Verification items for the finished model (mm, model axes). A direction names the side the tool comes from. Round coordinates to 2 decimals unless told otherwise and drop trailing zeros. Write each loop counter-clockwise with the first axis right and the second up, starting at its lowest first coordinate (ties: lowest second). Pieces come first, ordered by that corner, then holes. Notation, with made-up numbers: (51, 6.25) - (95, 6.25) arc R28 ccw to (95, 31.25) - close; hole circle Ø2 at (60, -6). An arc over 180 degrees is marked (long way). Answer as a JSON object with one key per item and string values.
```python
from build123d import *

# Parameters (mm, degrees)
BOSS_EXTRUDE1_DEPTH = 2.54
SKETCH6_W           = 5
SKETCH6_H           = 2.5
CUT_EXTRUDE2_DEPTH  = 0.2


with BuildPart() as part:
    # Sketch3 → Boss-Extrude1 (new body)
    with BuildSketch(Plane(origin=(0, 0, 0), x_dir=(1, 0, 0), z_dir=(0, 1, 0))):
        with BuildLine():
            ThreePointArc((-91.6492325, -96.833825344), (-94.514268143, 0.78027625), (-91.6492325, 98.394377843))
            ThreePointArc((-91.6492325, 98.394377843), (-77.728790436, 116.300836492), (-57.46959223, 126.498133029))
            ThreePointArc((-57.46959223, 126.498133029), (0, 128.705492461), (57.46959223, 126.498133029))
            ThreePointArc((57.46959223, 126.498133029), (77.728790436, 116.300836492), (91.6492325, 98.394377843))
            ThreePointArc((91.6492325, 98.394377843), (94.514268143, 0.78027625), (91.6492325, -96.833825344))
            ThreePointArc((91.6492325, -96.833825344), (77.728790436, -114.740283992), (57.46959223, -124.937580529))
            ThreePointArc((57.46959223, -124.937580529), (0, -127.144939961), (-57.46959223, -124.937580529))
            ThreePointArc((-57.46959223, -124.937580529), (-77.728790436, -114.740283992), (-91.6492325, -96.833825344))
        make_face()
    extrude(amount=BOSS_EXTRUDE1_DEPTH)

    # Sketch6 → Cut-Extrude2 (cut)
    with BuildSketch(Plane.XZ):
        Polygon((-80.884003768, 97.161784557), (-83.675257034, 101.310146306), (-81.601076159, 102.705772939), (-78.809822893, 98.55741119), align=None)
        Polygon((-60.2566864, 111.041014588), (-63.047939666, 115.189376338), (-65.122120541, 113.793749705), (-62.330867275, 109.645387955), align=None)
        Polygon((-67.644809829, 81.963964192), (-69.718990703, 80.568337559), (-72.510243969, 84.716699309), (-70.436063095, 86.112325942), align=None)
        Polygon((-51.16585421, 93.051940957), (-49.091673336, 94.44756759), (-51.882926602, 98.59592934), (-53.957107476, 97.200302707), align=None)
        Polygon((51.882926602, 98.59592934), (53.957107476, 97.200302707), (51.16585421, 93.051940957), (49.091673336, 94.44756759), align=None)
        Polygon((65.122120541, 113.793749705), (62.330867275, 109.645387955), (60.2566864, 111.041014588), (63.047939666, 115.189376338), align=None)
        Polygon((67.644809829, 81.963964192), (69.718990703, 80.568337559), (72.510243969, 84.716699309), (70.436063095, 86.112325942), align=None)
        Polygon((80.884003768, 97.161784557), (83.675257034, 101.310146306), (81.601076159, 102.705772939), (78.809822893, 98.55741119), align=None)
        with Locations((67.276236393, 10.46972375)):
            Rectangle(SKETCH6_W, SKETCH6_H)
        with Locations((87.276236393, 10.46972375)):
            Rectangle(SKETCH6_W, SKETCH6_H)
        with Locations((67.276236393, -12.03027625)):
            Rectangle(SKETCH6_W, SKETCH6_H)
        with Locations((87.276236393, -12.03027625)):
            Rectangle(SKETCH6_W, SKETCH6_H)
        Polygon((72.510243969, -86.277251808), (70.436063095, -87.672878441), (67.644809829, -83.524516692), (69.718990703, -82.128890059), align=None)
        Polygon((81.601076159, -104.266325439), (78.809822893, -100.11796369), (80.884003768, -98.722337057), (83.675257034, -102.870698806), align=None)
        Polygon((60.2566864, -112.601567088), (63.047939666, -116.749928837), (65.122120541, -115.354302204), (62.330867275, -111.205940455), align=None)
        Polygon((51.16585421, -94.612493457), (49.091673336, -96.00812009), (51.882926602, -100.15648184), (53.957107476, -98.760855207), align=None)
        Polygon((-65.122120541, -115.354302204), (-62.330867275, -111.205940455), (-60.2566864, -112.601567088), (-63.047939666, -116.749928837), align=None)
        Polygon((-51.882926602, -100.15648184), (-53.957107476, -98.760855207), (-51.16585421, -94.612493457), (-49.091673336, -96.00812009), align=None)
        Polygon((-80.884003768, -98.722337057), (-83.675257034, -102.870698806), (-81.601076159, -104.266325439), (-78.809822893, -100.11796369), align=None)
        Polygon((-67.644809829, -83.524516692), (-69.718990703, -82.128890059), (-72.510243969, -86.277251808), (-70.436063095, -87.672878441), align=None)
        with Locations((-67.276236393, 10.46972375)):
            Rectangle(SKETCH6_W, SKETCH6_H)
        with Locations((-67.276236393, -12.03027625)):
            Rectangle(SKETCH6_W, SKETCH6_H)
        with Locations((-87.276236393, -12.03027625)):
            Rectangle(SKETCH6_W, SKETCH6_H)
        with Locations((-87.276236393, 10.46972375)):
            Rectangle(SKETCH6_W, SKETCH6_H)
    extrude(amount=-CUT_EXTRUDE2_DEPTH, mode=Mode.SUBTRACT)


solid = part.part
```
1. Cross-section at B-B (z = -79.5). Record the boundary of the cut face in (x, y), plus the area to 3 significant figures.
Completed:
{"outline": "(-92.65, 0) - (92.65, 0) - (92.65, 2.54) - (-92.65, 2.54) - close", "area": "471 mm^2"}
2. Material ranges on probe 1 along Z at (x, y) = (-7, 1.1); probe 2 along X at (y, z) = (0.15, -8.5); probe 3 along Z at (x, y) = (-82.5, 1.9), recorded low to high. Write a range as from..to.
Completed:
{"probe 1": "z = -128.67..127.11", "probe 2": "x = -94.5..94.5", "probe 3": "z = -111.84..110.28"}
3. Go/stop test with flat-tipped pins: pin 1 (1 mm diameter, centred on y = 1.5, z = -45.5, fed in from +X); pin 2 (1.2 mm diameter, centred on x = -66, z = 10.5, fed in from -Y); pin 3 (1.5 mm diameter, centred on x = -46.5, y = 0.5, fed in from -Z). Record where each tip stops, or that it passes through.
Completed:
{"pin 1": "stops at x = 93.93", "pin 2": "stops at y = 0.2", "pin 3": "stops at z = -127.31"}
4. Mould release check, pull along Z, two halves, no side actions. Record for faces 3 (the face through (-77.481, 1.252, 114.943)), 4 (the face through (-77.975, 1.252, -116.097)), 5 (the face through (-70, 0.2, -85)): released by +Z, released by -Z, zero draft, split by the parting line, or undercut.
Completed:
{"face 3": "released by +Z", "face 4": "released by -Z", "face 5": "undercut"}
5. Access from +Z, -Z, +X, -X, +Y, -Y to the whole of each face (thin tool, end or side, straight path). Record for faces 1 (the face through (1, 0, -3)), 2 (the face through (70, 0.2, 83)).
Completed:
{"face 1": "+Z, -Z, +X, -X, -Y", "face 2": "-Y"}
6. Cross-section at A-A (y = 1.05). Record the boundary of the cut face in (x, z).
Completed:
{"outline": "(-91.65, -98.39) arc R51.54 ccw to (-57.47, -126.5) arc R749.23 ccw to (57.47, -126.5) arc R51.54 ccw to (91.65, -98.39) arc R1664.33 ccw to (91.65, 96.83) arc R51.54 ccw to (57.47, 124.94) arc R749.23 ccw to (-57.47, 124.94) arc R51.54 ccw to (-91.65, 96.83) arc R1664.33 ccw to start"}
